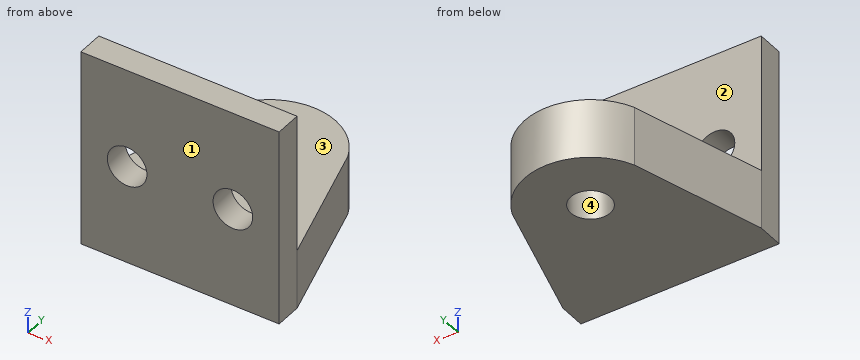
```python
from build123d import *

# Parameters (mm, degrees)
SKETCH7_W           = 15
SKETCH7_H           = 7.5
BOSS_EXTRUDE2_DEPTH = 2
SKETCH8_R           = 1.5
BOSS_EXTRUDE3_DEPTH = 4.5
SKETCH9_R           = 1.5
CUT_EXTRUDE1_DEPTH  = 3


with BuildPart() as part:
    # Sketch7 → Boss-Extrude2 (new body)
    with BuildSketch(Plane(origin=(0, 0, 0), x_dir=(1, 0, 0), z_dir=(0, 1, 0))):
        with Locations((0, -3.75)):
            Rectangle(SKETCH7_W, SKETCH7_H)
    boss_extrude2 = extrude(amount=BOSS_EXTRUDE2_DEPTH)

    # Sketch8 → Boss-Extrude3 (add)
    with BuildSketch(Plane(origin=(0, 0, 0), x_dir=(-1, 0, 0), z_dir=(0, 0, -1))):
        with BuildLine():
            Line((-4.598991345, 11.961957852), (-7.5, 2))
            Line((-7.5, 2), (7.5, 2))
            Line((7.5, 2), (4.615024569, 11.923940807))
            ThreePointArc((4.615024569, 11.923940807), (0.020629833, 14.999957441), (-4.598991345, 11.961957852))
        make_face()
        with Locations((0, 10)):
            Circle(SKETCH8_R, mode=Mode.SUBTRACT)
    extrude(amount=-BOSS_EXTRUDE3_DEPTH)

    # Mirror1: Boss-Extrude2 across plane
    add(boss_extrude2.mirror(Plane(origin=(7.5, 2, 7.5), x_dir=(1, 0, 0), z_dir=(0, 0, -1))))

    # Sketch9 → Cut-Extrude1 (cut, through all)
    with BuildSketch(Plane(origin=(0, 2, 0), x_dir=(1, 0, 0), z_dir=(0, 1, 0))):
        with Locations((4, -7.5)):
            Circle(SKETCH9_R)
    cut_extrude1 = extrude(amount=-CUT_EXTRUDE1_DEPTH, mode=Mode.SUBTRACT)

    # Mirror2: Cut-Extrude1 across plane
    add(cut_extrude1.mirror(Plane(origin=(0, 0, 0), x_dir=(0, 0, 1), z_dir=(1, 0, 0))), mode=Mode.SUBTRACT)


solid = part.part
```
Part model, mm, in its own coordinate system. Face numbers are marked on the shaded views. Round coordinates to 2 decimals unless told otherwise and drop trailing zeros. Write each loop counter-clockwise with the first axis right and the second up, starting at its lowest first coordinate (ties: lowest second). Pieces come first, ordered by that corner, then holes.
Item 1: Drop flat-ended pins along their axis: pin 1 Ø5 at (x, y) = (0, 10) entering from -Z; pin 2 Ø6 at (x, y) = (-2, 6.5) entering from +Z; pin 3 Ø5 at (x, z) = (-1, 10.5) entering from +Y. Give the stop position or say it passes through.
Results:
pin 1: stops at z = 0
pin 2: stops at z = 4.5
pin 3: stops at y = 2
Item 2: Cut at B-B, the plane x = 0. Give the cut face in (y, z).
Results:
outline: (0, 0) - (8.5, 0) - (8.5, 4.5) - (2, 4.5) - (2, 15) - (0, 15) - close; (11.5, 0) - (15, 0) - (15, 4.5) - (11.5, 4.5) - close
Item 3: Probe L1, parallel to X at y = 1.1, z = 7.5; L2, parallel to Z at x = -4, y = 0.5; L3, parallel to Z at x = 2.5, y = 13.25. List the from-to ranges inside material, lowest first.
Results:
L1: x = -7.5 to -5.5, -2.5 to 2.5, 5.5 to 7.5
L2: z = 0 to 6, 9 to 15
L3: z = 0 to 4.5
Item 4: Cut at C-C, the plane z = 7.5. Give the cut face in (x, y).
Results:
outline: (-7.5, 0) - (-5.5, 0) - (-5.5, 2) - (-7.5, 2) - close; (-2.5, 0) - (2.5, 0) - (2.5, 2) - (-2.5, 2) - close; (5.5, 0) - (7.5, 0) - (7.5, 2) - (5.5, 2) - close
Item 5: Cut at A-A, the plane z = 3. Give the cut face in (x, y), plus the area to 3 significant figures.
Results:
outline: (-7.5, 0) - (7.5, 0) - (7.5, 2) - (4.6, 11.96) arc R5 ccw to (-4.62, 11.92) - (-7.5, 2) - close; hole circle Ø3 at (0, 10)
area: 164 mm2
Item 6: Cut at D-D, the plane y = 10. Give the cut face in (x, z), plus the area to 3 significant figures.
Results:
outline: (-5.17, 0) - (-1.5, 0) - (-1.5, 4.5) - (-5.17, 4.5) - close; (1.5, 0) - (5.17, 0) - (5.17, 4.5) - (1.5, 4.5) - close
area: 33.1 mm2
Item 7: Two-plate mould, pull along Y, no slides. Class the marked faces 1, 2, 3 and 4: +Y half, -Y half, draft (parallel to the pull), parting line (faces both ways), or undercut.
Results:
face 1: -Y half
face 2: +Y half
face 3: draft
face 4: undercut
